from build123d import *

# Parameters (mm, degrees)
F0_R     = 3.923916639
F1_DEPTH = 15
F2_R     = 5
F2_R_2   = 4.99999


# Not quite as in the source:
# - a fillet or chamfer is up to 0.001 mm smaller than in the source, because OpenCascade refuses the exact size


with BuildPart() as f1:
    # F0 (on Right) → F1 (new body, symmetric)
    with BuildSketch(Plane.YZ):
        Polygon((0, 30), (0, 0), (150, 0), (150, 50), (65, 50), (65, 70), (40, 70), align=None)
        with Locations((25, 8)):
            Circle(F0_R, mode=Mode.SUBTRACT)
        with Locations((120, 8)):
            Circle(F0_R, mode=Mode.SUBTRACT)
        Polygon((44.1421356237, 60), (55, 60), (55, 35), (19.1421356237, 35), align=None, mode=Mode.SUBTRACT)
    extrude(amount=F1_DEPTH, both=True)

    # F2 (call 1 of 7: OpenCascade refuses the feature's edges together)
    f2_edges = [f1.edges().sort_by_distance(p)[0] for p in [
        (15, 52.5, 70),
        (0, 40, 70),
        (-15, 52.5, 70),
    ]]
    fillet(f2_edges, radius=F2_R)

    # F2#2 (call 2 of 7)
    f2_2_edges = [f1.edges().sort_by_distance(p)[0] for p in [
        (0, 0, 30),
    ]]
    fillet(f2_2_edges, radius=F2_R)

    # F2#3 (call 3 of 7)
    f2_3_edges = [f1.edges().sort_by_distance(p)[0] for p in [
        (0, 0, 0),
    ]]
    fillet(f2_3_edges, radius=F2_R)

    # F2#4 (call 4 of 7)
    f2_4_edges = [f1.edges().sort_by_distance(p)[0] for p in [
        (0, 150, 50),
    ]]
    fillet(f2_4_edges, radius=F2_R)

    # F2#5 (call 5 of 7) (radius 5 in the source; OpenCascade refuses exactly that, so slightly less here)
    f2_5_edges = [f1.edges().sort_by_distance(p)[0] for p in [
        (-15, 37.071068, 35),
        (-15, 55, 47.5),
        (-15, 49.571068, 60),
        (-15, 31.642136, 47.5),
    ]]
    fillet(f2_5_edges, radius=F2_R_2)

    # F2#6 (call 6 of 7)
    f2_6_edges = [f1.edges().sort_by_distance(p)[0] for p in [
        (15, 37.071068, 35),
        (15, 55, 47.5),
        (15, 31.642136, 47.5),
    ]]
    fillet(f2_6_edges, radius=F2_R)

    # F2#7 (call 7 of 7)
    f2_7_edges = [f1.edges().sort_by_distance(p)[0] for p in [
        (0, 150, 0),
    ]]
    fillet(f2_7_edges, radius=F2_R)


solid = f1.part
For this review, take the finished solid that the model builds, in its own axes (mm). A direction names the side the tool comes from. Round coordinates to 2 decimals unless told otherwise and drop trailing zeros. Order: outer loops, then holes, each group sorted by start corner. A loop starts at its lowest first (then second) coordinate and runs counter-clockwise, first axis right, second up. Notation, with made-up numbers: M -25.75,-0.5 L 5.25,-0.5 A21 ccw 5.25,8.5 Z; hole C -7,87 d8. An arc over 180 degrees is marked long. Write each question's results on one line, items separated by ' | '. Start each with the question number.
1. Add section D-D (y = 102). State the section outline as (x, z) points.
2. Add section C-C (x = -3). State the section outline as (y, z) points.
3. Add section A-A (z = 8). State the section outline as (x, y) points.
4. Tool access review of faces 4 (the face through (0, 37, 35)), 5 (the face through (-14, 33, 33)), 6 (the face through (13.496, 30.327, 48.201)): name each direction out of +Z, -Z, +X, -X, +Y, -Y from which nothing blocks a thin tool from reaching the whole face with its end or side.
5. Draft analysis for pull direction Y (two halves, no side actions). For faces 1 (the face through (-14, 51, 62)), 2 (the face through (0, 149, 48)), 3 (the face through (13, 53, 69)), state which applies: pulls with the +Y half, pulls with the -Y half, needs draft (parallel to the pull), parting line crosses it, or undercut.
6. Add section B-B (y = 120). State the section outline as (x, z) points, then the cut area to 3 significant figures.
7. To check wall thickness, follow L1, parallel to Z at x = 6, y = 49.5; L2, parallel to Z at x = 8.5, y = 137; L3, parallel to Z at x = 3.75, y = 120. State the ranges of each line that lie inside material, in increasing order. Write a range as [from, to].
8. Clearance check with flat-ended pins moving along their axes: pin 1 Ø16 at (x, y) = (3, 40) entering from +Z; pin 2 Ø7 at (y, z) = (25, 8) entering from -X; pin 3 Ø8 at (x, z) = (-10.5, 61.5) entering from +Y; pin 4 Ø2 at (x, y) = (2, 71) entering from +Z. State where each tip first meets the part, or that it passes through.
Output values:
1) outline: M -15,0 L 15,0 L 15,50 L -15,50 Z
2) outline: M 0,5 A5 ccw 5,0 L 145,0 A5 ccw 150,5 L 150,45 A5 ccw 145,50 L 65,50 L 65,70 L 42.07,70 A5 ccw 38.54,68.54 L 1.46,31.46 A5 ccw 0,27.93 Z; hole M 19.14,35 L 55,35 L 55,60 L 44.14,60 Z; hole C 25,8 d7.85; hole C 120,8 d7.85
3) outline: M -15,0 L 15,0 L 15,21.08 L -15,21.08 Z; M -15,28.92 L 15,28.92 L 15,116.08 L -15,116.08 Z; M -15,123.92 L 15,123.92 L 15,150 L -15,150 Z
4) face 4: +X, -X | face 5: -X | face 6: +X
5) face 1: undercut | face 2: pulls with the +Y half | face 3: needs draft
6) outline: M -15,0 L 15,0 L 15,4.08 L -15,4.08 Z; M -15,11.92 L 15,11.92 L 15,50 L -15,50 Z | area: 1,260 mm^2
7) L1: [0, 35], [60, 70] | L2: [0, 50] | L3: [0, 4.08], [11.92, 50]
8) pin 1: z = 70 | pin 2: through | pin 3: y = 65 | pin 4: z = 50
